Input: part model. Units: mm. Frame: model coordinates. Face numbers are marked on the shaded views. A direction names the side the tool comes from. Round coordinates to 2 decimals unless told otherwise and drop trailing zeros. Loops run counter-clockwise (first coordinate to the right, second up) from the corner with the lowest first, then second, coordinate; pieces in that order, holes last. Notation, with made-up numbers: (-14.75, 59.5) -> (38.25, 59.5) arc R35 cw to (38.25, 95.5) -> close; hole circle Ø10 at (-3, -13). An arc over 180 degrees is marked (long way). Answer in a Markdown table with one row per item. Add a question column.
Q1. Section B-B, the plane x = 47.5. Output: boundary loops of the cut face in (y, z).
Q2. Reachability of the marked faces 4, 5, 6 and 7 from +Z, -Z, +X, -X, +Y, -Y: full face, straight path, thin tool, end or side. Return the list, or none.
Q3. Ray query, L1, parallel to Y at x = 49, z = 19; L2, parallel to Y at x = 34, z = 27.5; L3, parallel to Z at x = -0.5, y = -20. Return the intervals inside material, ascending. Write a range as from..to.
Q4. Pin query (flat end, axial travel): pin 1 (5 mm diameter, centred on y = -1, z = 23.5, fed in from -X); pin 2 (3 mm diameter, centred on x = 25.5, y = 10.5, fed in from -Z); pin 3 (7.5 mm diameter, centred on x = -18.5, z = 21.5, fed in from -Y); pin 4 (12.5 mm diameter, centred on y = 13.5, z = 18.5, fed in from +X). Return the tip coordinate at first contact, or that it passes through.
Q5. Section C-C, the plane z = 16. Output: boundary loops of the cut face in (x, y).
Q6. Mould query, pull axis X, two halves, no side actions, for the marked faces 1, 2 and 3. Classes: pulls with the +X half, pulls with the -X half, needs draft (parallel to the pull), parting line crosses it, or undercut.
Q7. Section A-A, the plane y = -16.5. Output: boundary loops of the cut face in (x, z).
Q8. Section D-D, the plane y = 12. Output: boundary loops of the cut face in (x, z).
```python
from build123d import *

# Parameters (mm, degrees)
F1_DEPTH = 6.35
F2_R     = 5.08
F4_DEPTH = 25.4
F5_R     = 5.08


with BuildPart() as f1:
    # F0 (on Top) → F1 (new body)
    with BuildSketch(Plane.XY):
        with BuildLine():
            Line((-31.073933, 38.1), (-57.15, 38.1))
            Line((-57.15, 38.1), (-57.15, -38.1))
            Line((-57.15, -38.1), (57.15, -38.1))
            Line((57.15, -38.1), (57.15, 38.1))
            Line((57.15, 38.1), (31.073933, 38.1))
            ThreePointArc((31.073933, 38.1), (0, 7.026067), (-31.073933, 38.1))
        make_face()
    extrude(amount=F1_DEPTH)

    # F2
    f2_edges = [f1.edges().sort_by_distance(p)[0] for p in [
        (-57.15, 38.1, 3.175),
        (57.15, 38.1, 3.175),
    ]]
    fillet(f2_edges, radius=F2_R)

    # F3 (on face) → F4 (join)
    with BuildSketch(Plane.XY.offset(6.35)):
        with BuildLine():
            Line((-31.073933, 38.1), (-36.83, 38.1))
            Line((-36.83, 38.1), (-36.83, 0))
            Line((-36.83, 0), (-52.07, 0))
            Line((-52.07, 0), (-52.07, -38.1))
            Line((-52.07, -38.1), (-46.398055, -38.1))
            Line((-46.398055, -38.1), (-46.398055, -19.961452))
            Line((-46.398055, -19.961452), (46.057381, -19.961452))
            Line((46.057381, -19.961452), (46.057381, -38.1))
            Line((46.057381, -38.1), (51.308, -38.1))
            Line((51.308, -38.1), (51.308, 0))
            Line((51.308, 0), (36.068, 0))
            Line((36.068, 0), (36.068, 38.1))
            Line((36.068, 38.1), (31.073933, 38.1))
            ThreePointArc((31.073933, 38.1), (0, 7.026067), (-31.073933, 38.1))
        make_face()
    extrude(amount=F4_DEPTH)

    # F5
    f5_edges = [f1.edges().sort_by_distance(p)[0] for p in [
        (36.068, 0, 19.05),
        (-36.83, 0, 19.05),
    ]]
    fillet(f5_edges, radius=F5_R)


solid = f1.part
```
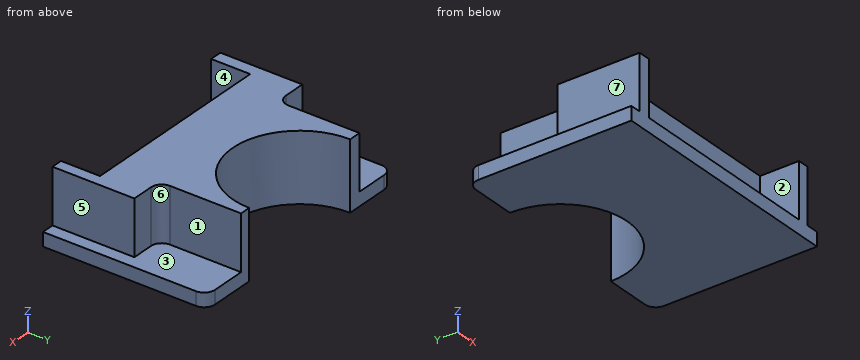
Answer block:
| question | item | result |
|---|---|---|
| 1 | outline | (-38.1, 0) -> (38.1, 0) -> (38.1, 6.35) -> (0, 6.35) -> (0, 31.75) -> (-38.1, 31.75) -> close |
| 2 | face 4 | +Z, -Y |
| 2 | face 5 | +Z, +X, +Y, -Y |
| 2 | face 6 | +Z, +X, +Y |
| 2 | face 7 | +Z, -X, +Y, -Y |
| 3 | L1 | -38.1..0 |
| 3 | L2 | -19.96..38.1 |
| 3 | L3 | 0..6.35 |
| 4 | pin 1 | x = -52.07 |
| 4 | pin 2 | z = 0 |
| 4 | pin 3 | y = -19.96 |
| 4 | pin 4 | x = 36.07 |
| 5 | outline | (-52.07, -38.1) -> (-46.4, -38.1) -> (-46.4, -19.96) -> (46.06, -19.96) -> (46.06, -38.1) -> (51.31, -38.1) -> (51.31, 0) -> (41.15, 0) arc R5.08 cw to (36.07, 5.08) -> (36.07, 38.1) -> (31.07, 38.1) arc R31.07 cw to (-31.07, 38.1) -> (-36.83, 38.1) -> (-36.83, 5.08) arc R5.08 cw to (-41.91, 0) -> (-52.07, 0) -> close |
| 6 | face 1 | pulls with the +X half |
| 6 | face 2 | undercut |
| 6 | face 3 | needs draft |
| 7 | outline | (-57.15, 0) -> (57.15, 0) -> (57.15, 6.35) -> (51.31, 6.35) -> (51.31, 31.75) -> (-52.07, 31.75) -> (-52.07, 6.35) -> (-57.15, 6.35) -> close |
| 8 | outline | (-57.15, 0) -> (-16.86, 0) -> (-16.86, 31.75) -> (-36.83, 31.75) -> (-36.83, 6.35) -> (-57.15, 6.35) -> close; (16.86, 0) -> (57.15, 0) -> (57.15, 6.35) -> (36.07, 6.35) -> (36.07, 31.75) -> (16.86, 31.75) -> close |
